Here's how the part is built. I have some questions about the finished solid (model axes, mm). Round coordinates to 2 decimals unless told otherwise and drop trailing zeros. Write each loop counter-clockwise with the first axis right and the second up, starting at its lowest first coordinate (ties: lowest second). Pieces come first, ordered by that corner, then holes. Notation, with made-up numbers: (41, 18.25) - (86, 18.25) arc R16 ccw to (86, 24.25) - close; hole circle Ø4 at (-7.5, 40.5). An arc over 180 degrees is marked (long way). One line per question, with ' | ' between items. Start each with the question number.
(1) Imagine slicing it at D-D (y = 8.25). Write out the boundary of the cut face in (x, z) (3 decimals).
(2) Imagine slicing it at A-A (x = 55.5). Write out the boundary of the cut face in (y, z) (3 decimals), plus the area to 3 significant figures.
(3) Imagine slicing it at B-B (z = -71.5). Write out the boundary of the cut face in (x, y), plus the area to 3 significant figures.
(4) Imagine slicing it at C-C (z = -203.2). Write out the boundary of the cut face in (x, y), plus the area to 3 significant figures.
(5) If I drill on L1, parallel to X at y = 2.5, z = -50.8; L2, parallel to Z at x = 163, y = 9 (3 decimals); L3, parallel to X at y = 0.5, z = -57, over which ranges is the centre line in solid material (lowest first)?
Autodesk Inventor part; units mm, degrees
ref_plane "YZ Plane" through (0, 0, 0) normal (1, 0, 0) x (0, 1, 0)
ref_plane "XZ Plane" through (0, 0, 0) normal (0, 1, 0) x (-1, 0, 0)
ref_plane "XY Plane" through (0, 0, 0) normal (0, 0, 1) x (1, 0, 0)
sketch "Sketch1" plane through (0, 0, 0) normal (0, 1, 0) x (-1, 0, 0)
  line L0 (0, 0) -> (-254, 0)
  line L1 (-254, 0) -> (-254, -254)
  line L2 (-254, -254) -> (0, -254)
  line L3 (0, -254) -> (0, 0)
  line L4 (-19.05, -228.6) -> (-234.95, -228.6)
  line L5 (-234.95, -228.6) -> (-234.95, -25.4)
  line L6 (-234.95, -25.4) -> (-19.05, -25.4)
  line L7 (-19.05, -25.4) -> (-19.05, -228.6)
  point P0 (-127, -228.6)
  point P1 (-127, -254)
  point P2 (-234.95, -127)
  point P3 (-254, -127)
  dimension "d0" = 254
  dimension "d1" = 254
  dimension "d2" = 25.4
  dimension "d3" = 19.05
extrude "Extrusion1" add sketch "Sketch1" along normal blind 12.7
sketch "Sketch2" plane through (0, 12.7, 0) normal (0, 1, 0) x (1, 0, 0)
  line L0 (0, 254) -> (0, 0)
  line L1 (254, 0) -> (254, 254)
  line L2 (19.05, 228.6) -> (234.95, 228.6)
  line L3 (234.95, 25.4) -> (19.05, 25.4)
  point P0 (9.525, 50.8)
  point P1 (9.525, 203.2)
  point P2 (244.475, 203.2)
  point P3 (244.475, 50.8)
  dimension "d6" = 9.525
  dimension "d7" = 9.525
  dimension "d8" = 25.4
  dimension "d9" = 25.4
hole "Hole1" at (9.525, 12.7, -50.8) at (9.525, 12.7, -203.2) at (244.475, 12.7, -203.2) at (244.475, 12.7, -50.8) direction (0, -1, 0) diameter 8.4074 end through all
sketch "Sketch3" plane through (0, 12.7, 0) normal (0, 1, 0) x (1, 0, 0)
  line L0 (254, 244.475) -> (0, 244.475)
  line L1 (254, 244.475) -> (254, 254)
  line L2 (0, 254) -> (254, 254)
  line L3 (0, 244.475) -> (0, 254)
  line L4 (0, 9.525) -> (254, 9.525)
  line L5 (0, 9.525) -> (0, 0)
  line L6 (254, 0) -> (0, 0)
  line L7 (254, 9.525) -> (254, 0)
extrude "Extrusion2" cut sketch "Sketch3" against normal through all
properties part number "Smooth Rod Brace Bottom"
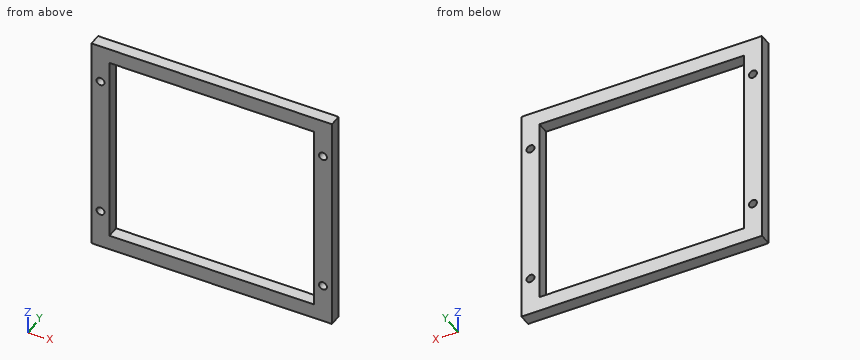
Check sheet entries:
1) outline: (0, -244.475) - (254, -244.475) - (254, -9.525) - (0, -9.525) - close; hole circle Ø8.407 at (9.525, -203.2); hole circle Ø8.407 at (9.525, -50.8); hole (19.05, -228.6) - (234.95, -228.6) - (234.95, -25.4) - (19.05, -25.4) - close; hole circle Ø8.407 at (244.475, -203.2); hole circle Ø8.407 at (244.475, -50.8)
2) outline: (0, -244.475) - (12.7, -244.475) - (12.7, -228.6) - (0, -228.6) - close; (0, -25.4) - (12.7, -25.4) - (12.7, -9.525) - (0, -9.525) - close | area: 403 mm^2
3) outline: (0, 0) - (19.05, 0) - (19.05, 12.7) - (0, 12.7) - close; (234.95, 0) - (254, 0) - (254, 12.7) - (234.95, 12.7) - close | area: 484 mm^2
4) outline: (0, 0) - (5.32, 0) - (5.32, 12.7) - (0, 12.7) - close; (13.73, 0) - (19.05, 0) - (19.05, 12.7) - (13.73, 12.7) - close; (234.95, 0) - (240.27, 0) - (240.27, 12.7) - (234.95, 12.7) - close; (248.68, 0) - (254, 0) - (254, 12.7) - (248.68, 12.7) - close | area: 270 mm^2
5) L1: 0 to 5.32, 13.73 to 19.05, 234.95 to 240.27, 248.68 to 254 | L2: -244.475 to -228.6, -25.4 to -9.525 | L3: 0 to 19.05, 234.95 to 254
